Input: dimensioned drawing with shaded views. Units: mm. Origin: part minimum x, y, z. A direction names the side the tool comes from. Give positions to 0.01 mm unless a question says otherwise; leave off trailing zeros. Write each loop counter-clockwise with the first axis right and the second up, starting at its lowest first coordinate (ties: lowest second). Pieces come first, ordered by that corner, then holes. Notation, with made-up numbers: (70.25, 13.5) -> (75.25, 13.5) arc R23 cw to (75.25, 32.5) -> close; hole circle Ø11 at (-6.75, -36). An arc over 180 degrees is marked (long way). Answer in a Markdown table with one row per item. Add a question column.
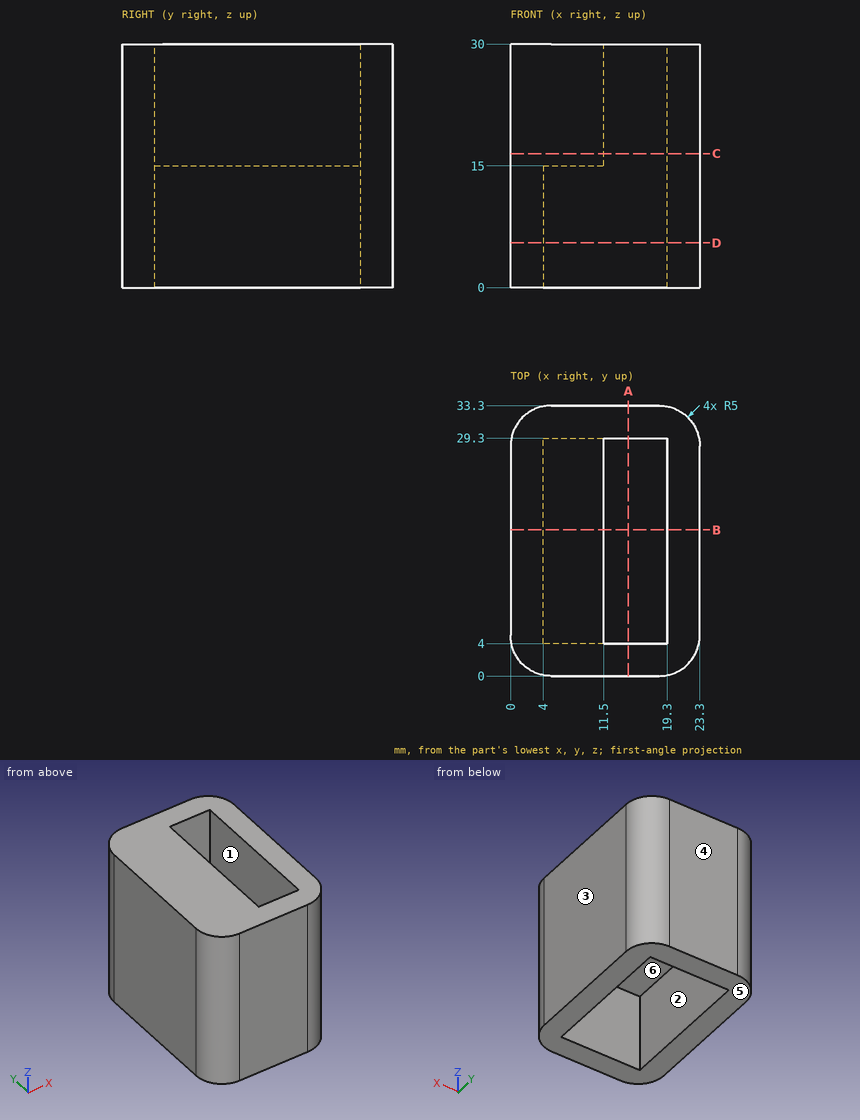
Q1. Pull-direction query (Y, two-part tool) for the marked faces 4, 5 and 6; classes: +Y half, -Y half, draft (parallel to the pull), parting line (faces both ways), or undercut.
Q2. Line query: probe 1 along X at (y, z) = (8, 18.25); probe 2 along Y at (x, z) = (12, 8.75); probe 3 along X at (y, z) = (16.5, 9.75). Output: solid intervals per line, ascending. Write a range as from..to.
Q3. Contact query for a flat-ended pin moving along its axis: pin 1 Ø2 at (x, y) = (7, 14.5) entering from -Z. Output: stop coordinate, or through.
Q4. Section D-D on z = 5.5. Return loops of the section in (x, y).
Q5. Access query for the marked faces 1, 2 and 3. Directions: +Z, -Z, +X, -X, +Y, -Y. A direction counts if a zero-diameter tool reaches every point of the face in a straight line with its end or side. Return the directions, or none.
Q6. Section C-C on z = 16.5. Return loops of the section in (x, y).
Q7. Section B-B on y = 18. Return loops of the section in (x, z).
Q8. Section A-A on x = 14.5. Return loops of the section in (y, z), and give its area (3 significant figures).
Checks:
| question | item | result |
|---|---|---|
| 1 | face 4 | +Y half |
| 1 | face 5 | draft |
| 1 | face 6 | undercut |
| 2 | probe 1 | 0..11.5, 19.3..23.3 |
| 2 | probe 2 | 0..4, 29.3..33.3 |
| 2 | probe 3 | 0..4, 19.3..23.3 |
| 3 | pin 1 | z = 15 |
| 4 | outline | (0, 5) arc R5 ccw to (5, 0) -> (18.3, 0) arc R5 ccw to (23.3, 5) -> (23.3, 28.3) arc R5 ccw to (18.3, 33.3) -> (5, 33.3) arc R5 ccw to (0, 28.3) -> close; hole (4, 4) -> (19.3, 4) -> (19.3, 29.3) -> (4, 29.3) -> close |
| 5 | face 1 | +Z, -Z |
| 5 | face 2 | -Z |
| 5 | face 3 | +Z, -Z, +X, +Y, -Y |
| 6 | outline | (0, 5) arc R5 ccw to (5, 0) -> (18.3, 0) arc R5 ccw to (23.3, 5) -> (23.3, 28.3) arc R5 ccw to (18.3, 33.3) -> (5, 33.3) arc R5 ccw to (0, 28.3) -> close; hole (11.5, 4) -> (19.3, 4) -> (19.3, 29.3) -> (11.5, 29.3) -> close |
| 7 | outline | (0, 0) -> (4, 0) -> (4, 15) -> (11.5, 15) -> (11.5, 30) -> (0, 30) -> close; (19.3, 0) -> (23.3, 0) -> (23.3, 30) -> (19.3, 30) -> close |
| 8 | outline | (0, 0) -> (4, 0) -> (4, 30) -> (0, 30) -> close; (29.3, 0) -> (33.3, 0) -> (33.3, 30) -> (29.3, 30) -> close |
| 8 | area | 240 mm^2 |
